Autodesk Inventor part; units mm, degrees
ref_plane "YZ Plane" through (0, 0, 0) normal (1, 0, 0) x (0, 1, 0)
ref_plane "XZ Plane" through (0, 0, 0) normal (0, 1, 0) x (-1, 0, 0)
ref_plane "XY Plane" through (0, 0, 0) normal (0, 0, 1) x (1, 0, 0)
sketch "스케치1" plane through (0, 0, 0) normal (0, 1, 0) x (-1, 0, 0)
  circle A0 centre (0, 0) radius 47
  circle A1 centre (0, 0) radius 35
  line L0 (0, 0) -> (0, 145.5)
  circle A2 centre (0, 145.5) radius 48.5
  circle A3 centre (0, 145.5) radius 36.5
  dimension "d0" = 94
  dimension "d1" = 12
  dimension "d2" = 145.5
  dimension "d3" = 97
  dimension "d4" = 12
extrude "돌출1" add sketch "스케치1" along normal blind 30 contours A0
sketch "스케치2" plane through (0, 30, 0) normal (0, 1, 0) x (1, 0, 0)
  line L0 (-55, 60) -> (55, 60)
  line L1 (55, 60) -> (55, -60)
  line L2 (55, -60) -> (-55, -60)
  line L3 (-55, -60) -> (-55, 60)
  line L4 (-55, 60) -> (55, -60) construction
  line L5 (55, 60) -> (-55, -60) construction
  point P0 (0, 0)
  dimension "d7" = 110
  dimension "d8" = 120
extrude "돌출2" add sketch "스케치2" along normal blind 20
fillet "모깎기1" radius 15 2 edges at (-55, 40, -60) (55, 40, -60)
sketch "스케치5" plane through (0, 50, 0) normal (0, 1, 0) x (1, 0, 0)
  circle A0 centre (0, 0) radius 30
  circle A1 centre (0, 0) radius 38
  dimension "d22" = 60
  dimension "d23" = 8
extrude "돌출5" [suppressed]
sketch "스케치6" plane through (0, 50, 0) normal (0, 1, 0) x (1, 0, 0)
  circle A0 centre (0, 0) radius 30
extrude "돌출6" cut sketch "스케치6" against normal blind 15
sketch "스케치7" plane through (0, 50, 0) normal (0, 1, 0) x (1, 0, 0)
  line L0 (-55, 45) -> (-55, -60)
  line L1 (-55, -60) -> (0, -91.7543)
  line L2 (-55, -60) -> (8.5085, -60) construction
  line L3 (55, -60) -> (55, 45)
  line L4 (0, -91.7543) -> (55, -60)
  line L5 (0, -91.7543) -> (0, -76.7543)
  circle A0 centre (0, -76.7543) radius 8.25
  line L6 (-55, -60) -> (55, -60)
  point P0 (0, 0)
  dimension "d28" = 30
  dimension "d29" = 15
  dimension "d30" = 16.5
extrude "돌출7" add sketch "스케치7" against normal blind 10
fillet "모깎기2" radius 5 1 edges at (0, 45, 91.7543)
sketch "스케치8" plane through (0, 0, 0) normal (0, -1, 0) x (1, 0, 0)
  circle A0 centre (0, 0) radius 35
extrude "돌출8" add sketch "스케치8" against normal up to surface (30 mm away)
sketch "스케치9" plane through (0, 0, 0) normal (1, 0, 0) x (0, 1, 0)
  line L0 (0, -47) -> (0, 47)
  line L1 (0, 0) -> (0, 47)
  line L2 (0, 47) -> (0, 23.5)
  line L3 (0, 23.5) -> (2.056, 47)
  line L4 (0, 47) -> (30, 47)
  line L5 (0, 23.5) -> (23.5898, 23.5) construction
  line L6 (0, 0) -> (0, -47)
  line L7 (0, -23.5) -> (2.056, -47)
  line L8 (0, -47) -> (2.056, -47)
  dimension "d36" = 85
extrude "돌출9" cut sketch "스케치9" along normal mid plane 100
sketch "스케치10" plane through (0, 50, 0) normal (0, 1, 0) x (1, 0, 0)
  line L0 (-55, -60) -> (-2.5, -90.3109)
  line L1 (-55, -60) -> (-2.5, -90.3109)
  line L2 (-2.5, -90.3109) -> (0, -91.7543)
  line L3 (0, -91.7543) -> (-55, -91.7543)
  line L4 (-55, -91.7543) -> (-55, -60)
  line L5 (55, -60) -> (2.5, -90.3109)
  line L6 (0, -91.7543) -> (2.5, -90.3109)
  arc A0 (-2.5, -90.3109) -> (2.5, -90.3109) centre (0, -85.9808) ccw
  circle A1 centre (0, -85.9808) radius 5
  point P0 (0, 0)
  dimension "d41" = 31.7543
  dimension "d42" = 55
  dimension "d43" = 60.6218
extrude "돌출10" add sketch "스케치10" against normal up to surface (10 mm away) contours L0 L2 L3 L4 | A0 L6 L2
properties part number "bracket_2"
Work out the finished part from the listing and answer in its coordinate system (mm). A direction names the side the tool comes from. Round coordinates to 2 decimals unless told otherwise and drop trailing zeros. Loops run counter-clockwise (first coordinate to the right, second up) from the corner with the lowest first, then second, coordinate; pieces in that order, holes last.
(1) The part is cut by section D-D, the plane z = 78.5. Give the vertices of the cut face in (x, y), and give its area (3 significant figures).
Computed values:
outline: (-55, 40) - (-8.06, 40) - (-8.06, 50) - (-55, 50) - close; (8.06, 40) - (22.96, 40) - (22.96, 50) - (8.06, 50) - close
area: 618 mm2
(2) Each of these flat-tipped pins is pushed along its axis until it touches: P1, Ø3, axis at x = 14.5, y = 33, coming from the +Z side; P2, Ø1.5, axis at y = 9, z = 33, coming from the -X side; P3, Ø5, axis at y = 14.5, z = 26, coming from the -X side; P4, Ø10, axis at x = 7, z = -13, coming from the -Y side. Where does it stop, or does it pass through?
Computed values:
P1: stops at z = 60
P2: stops at x = -34.19
P3: stops at x = -40.7
P4: stops at y = 0
(3) The part is cut by section B-B, the plane y = 38. Give the vertices of the cut face in (x, z).
Computed values:
outline: (-55, -45) arc R15 ccw to (-40, -60) - (40, -60) arc R15 ccw to (55, -45) - (55, 60) - (-55, 60) - close; hole circle Ø60 at (0, 0)
(4) The part is cut by section C-C, the plane x = 15.5. Give the vertices of the cut face in (y, z), and give its area (3 significant figures).
Computed values:
outline: (0, -23.5) - (1.83, -44.37) - (30, -44.37) - (30, -60) - (50, -60) - (50, -25.69) - (35, -25.69) - (35, 25.69) - (50, 25.69) - (50, 82.81) - (40, 82.81) - (40, 60) - (30, 60) - (30, 44.37) - (1.83, 44.37) - (0, 23.5) - close
area: 4,480 mm2
(5) For faces 1 (the flat face through (-13, 40, 72)), 2 (the cylindrical face through (-29.97, 42.6, -1.32)), 3 (the flat face through (-25, 30, -41)), 4 (the cylindrical face through (4.44, 45.07, 69.8)), determine the directions among +Z, -Z, +X, -X, +Y, -Y from which every point of the face is accessible in a straight line to the end or side of a thin tool.
Computed values:
face 1: +Z, +X, -X, -Y
face 2: +Y
face 3: -Y
face 4: +Y, -Y
(6) The part is cut by section A-A, the plane z = 0. Give the vertices of the cut face in (x, y).
Computed values:
outline: (-55, 30) - (-47, 30) - (-47, 0) - (47, 0) - (47, 30) - (55, 30) - (55, 50) - (30, 50) - (30, 35) - (-30, 35) - (-30, 50) - (-55, 50) - close
(7) Find the intervals of material crossed by L1, parallel to Z at x = 0, y = 43.25; L2, parallel to X at y = 43.5, z = 0; L3, parallel to Z at x = 0, y = 38.5, in increasing order.
Computed values:
L1: z = -60 to -30, 30 to 68.5, 85 to 91.75
L2: x = -55 to -30, 30 to 55
L3: z = -60 to -30, 30 to 60
